from build123d import *
from OCP.BRepFilletAPI import BRepFilletAPI_MakeChamfer

# Parameters (mm, degrees)
RESSALTO_EXTRUS_O1_DEPTH = 13
ESBO_O2_W                = 15
ESBO_O2_H                = 6
ESBO_O2_W_2              = 4
ESBO_O2_H_2              = 16
RESSALTO_EXTRUS_O2_DEPTH = 15
ESBO_O3_R                = 1
CORTE_EXTRUS_O1_DEPTH    = 77.870020164
ESBO_O10_R               = 1.7
CORTE_EXTRUS_O4_DEPTH    = 10
ESBO_O11_W               = 25
ESBO_O11_H               = 34.7
CORTE_EXTRUS_O5_DEPTH    = 10
RESSALTO_EXTRUS_O3_DEPTH = 17
RESSALTO_EXTRUS_O4_REACH = 77.374
ESBO_O7_W                = 4
ESBO_O7_H                = 5
ESBO_O8_W                = 15
ESBO_O8_H                = 3.5
RESSALTO_EXTRUS_O5_DEPTH = 2.5
CHANFRO2_SIZE            = 2
CHANFRO2_SIZE_2          = 7
CHANFRO3_SIZE            = 1.5
CHANFRO3_SIZE2           = 3.216760381
ESBO_O12_W               = 12.6
ESBO_O12_H               = 10.6
CORTE_EXTRUS_O6_DEPTH    = 10
CORTE_EXTRUS_O7_DEPTH    = 22
ESBO_O15_R               = 2
CORTE_EXTRUS_O9_DEPTH    = 15


with BuildPart() as part:
    # Esboço1 → Ressalto-extrusão1 (new body)
    with BuildSketch(Plane.XY):
        Polygon((-12.5, 0), (12.5, 0), (12.5, -40), (7.5, -70), (-7.5, -70), (-12.5, -40), align=None)
    extrude(amount=RESSALTO_EXTRUS_O1_DEPTH)

    # Esboço2 → Ressalto-extrusão2 (add)
    with BuildSketch(Plane.XY.offset(13)):
        with Locations((-5, -32.3)):
            Rectangle(ESBO_O2_W, ESBO_O2_H)
        with Locations((-5, -3)):
            Rectangle(ESBO_O2_W, ESBO_O2_H)
        with Locations((10.5, -12)):
            Rectangle(ESBO_O2_W_2, ESBO_O2_H_2)
    extrude(amount=RESSALTO_EXTRUS_O2_DEPTH)

    # Esboço3 → Corte-extrusão1 (cut, through all)
    with BuildSketch(Plane(origin=(2.5, 0, 0), x_dir=(0, 0, -1), z_dir=(1, 0, 0))):
        with Locations(Location((-20.5, -3.8, 0), (0, 0, 90))):
            Circle(ESBO_O3_R)
        with Locations(Location((-20.5, -31.5, 0), (0, 0, 270))):
            Circle(ESBO_O3_R)
    extrude(amount=-CORTE_EXTRUS_O1_DEPTH, mode=Mode.SUBTRACT)

    # Esboço10 → Corte-extrusão4 (cut)
    with BuildSketch(Plane(origin=(12.5, 0, 0), x_dir=(0, 0, -1), z_dir=(1, 0, 0))):
        with Locations((-20.5, -12)):
            Circle(ESBO_O10_R)
        with BuildLine():
            Line((-13, -4), (-28, -4))
            Line((-28, -4), (-28, -20))
            Line((-28, -20), (-13, -20))
            Line((-13, -20), (-21.684004699, -18.391254405))
            ThreePointArc((-21.684004699, -18.391254405), (-27, -12), (-21.684004699, -5.608745595))
            Line((-21.684004699, -5.608745595), (-13, -4))
        make_face()
    extrude(amount=-CORTE_EXTRUS_O4_DEPTH, mode=Mode.SUBTRACT)

    # Esboço11 → Corte-extrusão5 (cut)
    with BuildSketch(Plane.XY.offset(13)):
        with Locations((0, -52.65)):
            Rectangle(ESBO_O11_W, ESBO_O11_H)
    extrude(amount=-CORTE_EXTRUS_O5_DEPTH, mode=Mode.SUBTRACT)

    # Esboço6 → Ressalto-extrusão3 (add)
    with BuildSketch(Plane.XZ.offset(70)):
        Polygon((-5, 4), (-5, 7.5), (-4.75, 7.5), (-4.75, 10), (-7.5, 10), (-7.5, 3), (7.5, 3), (7.5, 10), (4.75, 10), (4.75, 7.5), (5, 7.5), (5, 4), align=None)
    extrude(amount=-RESSALTO_EXTRUS_O3_DEPTH)

    # Ressalto-extrusão4: up to this face of the body (flat: up to its plane)
    ressalto_extrus_o4_end = Plane(part.part.faces().sort_by_distance((-6.125, -61.5, 10))[0])
    # Esboço7 → Ressalto-extrusão4 (add, up to the picked face)
    with BuildSketch(Plane.XY.offset(3), mode=Mode.PRIVATE) as ressalto_extrus_o4_sk1:
        with Locations((0, -40.5)):
            Rectangle(ESBO_O7_W, ESBO_O7_H)
    ressalto_extrus_o4_tool1 = split(extrude(ressalto_extrus_o4_sk1.sketch, amount=RESSALTO_EXTRUS_O4_REACH, mode=Mode.PRIVATE), bisect_by=ressalto_extrus_o4_end, keep=Keep.BOTH, mode=Mode.PRIVATE)
    # Esboço7 → Ressalto-extrusão4 (add, up to the picked face)
    with BuildSketch(Plane.XY.offset(3), mode=Mode.PRIVATE) as ressalto_extrus_o4_sk2:
        with Locations((5.5, -55.5)):
            Rectangle(ESBO_O7_W, ESBO_O7_H)
    ressalto_extrus_o4_tool2 = split(extrude(ressalto_extrus_o4_sk2.sketch, amount=RESSALTO_EXTRUS_O4_REACH, mode=Mode.PRIVATE), bisect_by=ressalto_extrus_o4_end, keep=Keep.BOTH, mode=Mode.PRIVATE)
    # Esboço7 → Ressalto-extrusão4 (add, up to the picked face)
    with BuildSketch(Plane.XY.offset(3), mode=Mode.PRIVATE) as ressalto_extrus_o4_sk3:
        with Locations((-5.5, -55.5)):
            Rectangle(ESBO_O7_W, ESBO_O7_H)
    ressalto_extrus_o4_tool3 = split(extrude(ressalto_extrus_o4_sk3.sketch, amount=RESSALTO_EXTRUS_O4_REACH, mode=Mode.PRIVATE), bisect_by=ressalto_extrus_o4_end, keep=Keep.BOTH, mode=Mode.PRIVATE)
    add(ressalto_extrus_o4_tool1.solids().sort_by(Axis((0, -40.5, 3), (0, 0, 1)))[0])
    add(ressalto_extrus_o4_tool2.solids().sort_by(Axis((5.5, -55.5, 3), (0, 0, 1)))[0])
    add(ressalto_extrus_o4_tool3.solids().sort_by(Axis((-5.5, -55.5, 3), (0, 0, 1)))[0])

    # Esboço8 → Ressalto-extrusão5 (add)
    with BuildSketch(Plane.XY.offset(10)):
        with Locations((0, -68.25)):
            Rectangle(ESBO_O8_W, ESBO_O8_H)
        with Locations((0, -55.75)):
            Rectangle(ESBO_O8_W, ESBO_O8_H)
    extrude(amount=-RESSALTO_EXTRUS_O5_DEPTH)

    # Chanfro2
    chanfro2_edges_1 = [part.edges().sort_by_distance(p)[0] for p in [
        (7.5, -61.5, 3),
    ]]
    chanfro2_side_1 = [part.faces().sort_by_distance(p)[0] for p in [
        (7.54, -61.5, 3),
    ]]
    chanfro2_edges_2 = [part.edges().sort_by_distance(p)[0] for p in [
        (-7.5, -61.5, 3),
    ]]
    chanfro2_side_2 = [part.faces().sort_by_distance(p)[0] for p in [
        (-7.54, -61.5, 3),
    ]]
    chanfro2 = BRepFilletAPI_MakeChamfer(part.part.solid().wrapped)
    for e in chanfro2_edges_1:
        chanfro2.Add(CHANFRO2_SIZE - 0.0001, CHANFRO2_SIZE_2 - 0.0001, e.wrapped, chanfro2_side_1[0].wrapped)
    for e in chanfro2_edges_2:
        chanfro2.Add(CHANFRO2_SIZE - 0.0001, CHANFRO2_SIZE_2 - 0.0001, e.wrapped, chanfro2_side_2[0].wrapped)
    add(Compound.cast(chanfro2.Shape()), mode=Mode.REPLACE)  # a hair under: the kernel refuses the full size

    # Chanfro3
    chanfro3_edges = [part.edges().sort_by_distance(p)[0] for p in [
        (0, -70, 0),
    ]]
    chanfro3_side = [part.faces().sort_by_distance(p)[0] for p in [
        (7.319722436, -70, 9.99995),
    ]]
    chamfer(chanfro3_edges, length=CHANFRO3_SIZE, length2=CHANFRO3_SIZE2, reference=chanfro3_side[0])

    # Esboço12 → Corte-extrusão6 (cut)
    with BuildSketch(Plane(origin=(0, 0, 0), x_dir=(1, 0, 0), z_dir=(0, 1, 0))):
        with Locations((0, -6.5)):
            Rectangle(ESBO_O12_W, ESBO_O12_H)
    extrude(amount=-CORTE_EXTRUS_O6_DEPTH, mode=Mode.SUBTRACT)

    # Esboço13 → Corte-extrusão7 (cut)
    with BuildSketch(Plane(origin=(0, -10, 0), x_dir=(1, 0, 0), z_dir=(0, 1, 0))):
        with BuildLine():
            Line((-3.405877273, -11.8), (3.405877273, -11.8))
            ThreePointArc((3.405877273, -11.8), (6.3, -6.5), (3.405877273, -1.2))
            Line((3.405877273, -1.2), (-3.405877273, -1.2))
            ThreePointArc((-3.405877273, -1.2), (-6.3, -6.5), (-3.405877273, -11.8))
        make_face()
    extrude(amount=-CORTE_EXTRUS_O7_DEPTH, mode=Mode.SUBTRACT)

    # Esboço15 → Corte-extrusão9 (cut)
    with BuildSketch(Plane.ZY.offset(12.5)):
        with Locations((6, -28)):
            Circle(ESBO_O15_R)
    extrude(amount=-CORTE_EXTRUS_O9_DEPTH, mode=Mode.SUBTRACT)


solid = part.part
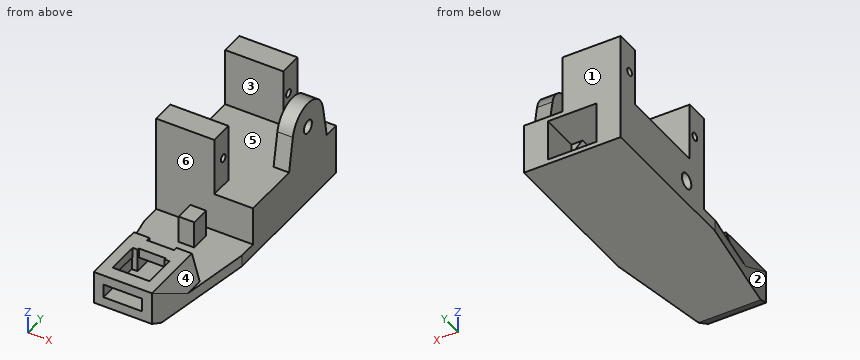
Design review of the part built by this model. Coordinates are the model's own, in mm. Face numbers are marked on the shaded views. A direction names the side the tool comes from. Give positions to 0.01 mm unless a question says otherwise; leave off trailing zeros. Write each loop counter-clockwise with the first axis right and the second up, starting at its lowest first coordinate (ties: lowest second). Pieces come first, ordered by that corner, then holes. Notation, with made-up numbers: M 85,-28.5 L 144,-28.5 A19 ccw 144,-15.5 Z; hole C 0,-9.75 d4. An arc over 180 degrees is marked long. Return JSON: item names as keys, results as strings. Group by question number.
Item 1: Take a section at B-B (z = 26.25). Give the boundary of the cut face in (x, y), plus the area to 3 significant figures.
Item 2: Take a section at A-A (y = -12). Give the boundary of the cut face in (x, z).
Item 3: Tool access review of the marked faces 4, 5 and 6: name each direction out of +Z, -Z, +X, -X, +Y, -Y from which nothing blocks a thin tool from reaching the whole face with its end or side.
Item 4: Clearance check with flat-ended pins moving along their axes: pin 1 Ø4 at (y, z) = (-55, 7) entering from -X; pin 2 Ø3.5 at (x, z) = (1.5, 5) entering from +Y; pin 3 Ø4 at (y, z) = (-40, 6) entering from +X; pin 4 Ø2 at (y, z) = (-45.5, 6) entering from +X (1 decimal). State where each tip first meets the part, or that it passes through.
Item 5: The part is to be moulded in two halves that separate along Y. For the marked faces 1, 2 and 3, say which applies: pulls with the +Y half, pulls with the -Y half, needs draft (parallel to the pull), parting line crosses it, or undercut.
Item 6: Take a section at D-D (y = -42). Give the boundary of the cut face in (x, z).
Item 7: Take a section at C-C (z = 17.25). Give the boundary of the cut face in (x, y), plus the area to 3 significant figures.
Item 8: Wall thickness on line 1 along Z through (x, y) = (-3, -3.8); line 2 along Z through (x, y) = (-7.5, -3.8); line 3 along Y through (x, z) = (-10.25, 6): over which ranges is each line inside the solid? List them lowest first.
Return value:
{
 "1": {"outline": "M -12.5,-35.3 L 2.5,-35.3 L 2.5,-29.3 L -12.5,-29.3 Z; M -12.5,-6 L 2.5,-6 L 2.5,0 L -12.5,0 Z; M 8.5,-15.03 L 12.5,-15.03 L 12.5,-8.97 L 8.5,-8.97 Z", "area": "204 mm2"},
 "2": {"outline": "M -12.5,0 L 12.5,0 L 12.5,18.8 L 8.5,18.8 L 8.5,13 L -12.5,13 Z; M 8.5,22.2 L 12.5,22.2 L 12.5,27 L 8.5,27 Z; hole M -3.41,1.2 L 3.41,1.2 A6.3 ccw 3.41,11.8 L -3.41,11.8 A6.3 ccw Z"},
 "3": {"face 4": "+Z, +X, -Y", "face 5": "+Z", "face 6": "+Z, +X, -X"},
 "4": {"pin 1": "stops at x = -8.93", "pin 2": "stops at y = -32", "pin 3": "stops at x = 2", "pin 4": "passes through"},
 "5": {"face 1": "pulls with the +Y half", "face 2": "pulls with the -Y half", "face 3": "undercut"},
 "6": {"outline": "M -12.17,0 L 12.17,0 L 12.17,3 L 2,3 L 2,10 L -2,10 L -2,3 L -12.17,3 Z"},
 "7": {"outline": "M -12.5,-35.3 L 2.5,-35.3 L 2.5,-29.3 L -12.5,-29.3 Z; M -12.5,-6 L 2.5,-6 L 2.5,0 L -12.5,0 Z; M 8.5,-19.21 L 12.5,-19.21 L 12.5,-4.79 L 8.5,-4.79 Z", "area": "238 mm2"},
 "8": {"line 1": "z = 0 to 1.2, 11.8 to 19.5, 21.5 to 28", "line 2": "z = 0 to 19.5, 21.5 to 28", "line 3": "y = -35.3 to -30, -26 to 0"}
}
